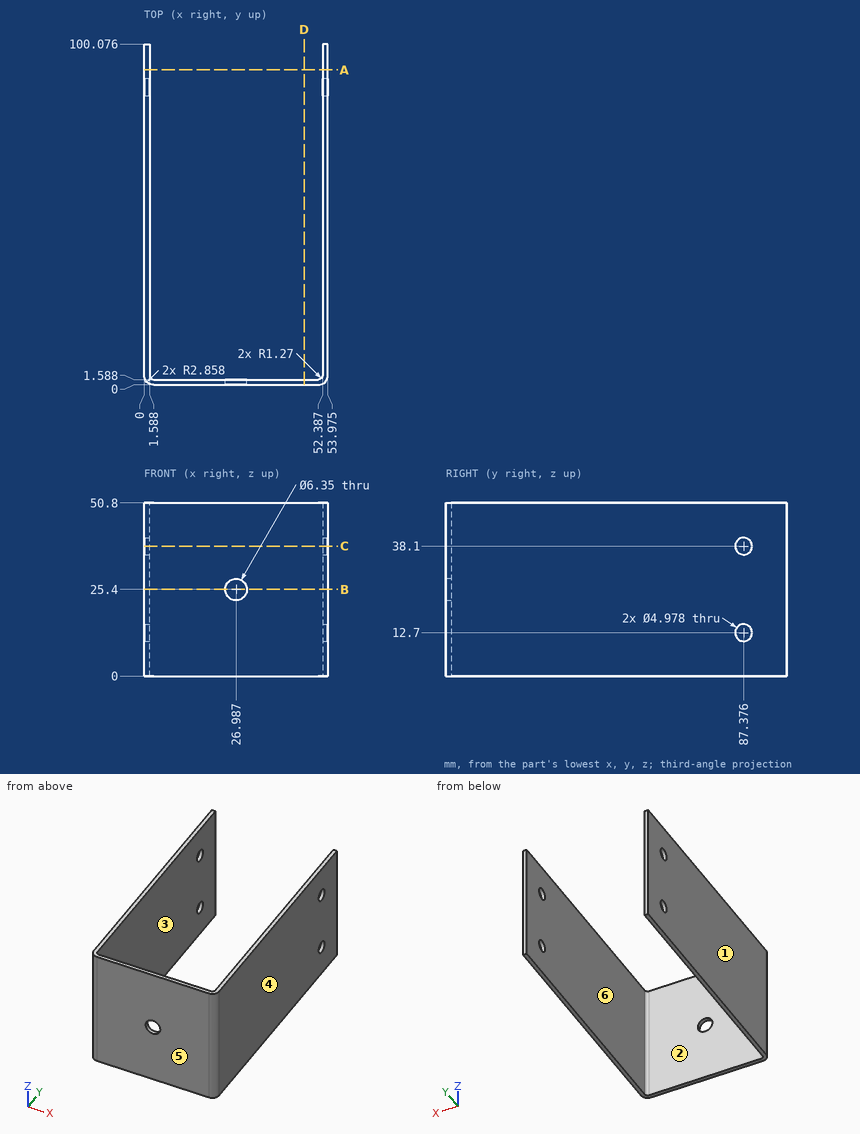
Print and shaded views of the part. All mm, measured from the part's lowest x, y and z. A direction names the side the tool comes from. Round coordinates to 2 decimals unless told otherwise and drop trailing zeros. Write each loop counter-clockwise with the first axis right and the second up, starting at its lowest first coordinate (ties: lowest second). Pieces come first, ordered by that corner, then holes.
(1) Slice it at C-C, the plane z = 38.1. Write the cut outline in (x, y) (1 decimal).
(2) Mould opens along X. For the marked faces 3, 4, 5 and 6 say: pulls with the +X half, pulls with the -X half, needs draft (parallel to the pull), parting line crosses it, or undercut.
(3) Probe line 1 along X through (y, z) = (17, 13.5) (1 decimal); line 2 along Y through (x, z) = (25.5, 47.5). List the from-to ranges inside material, lowest first.
(4) 3-axis set-ups, long thin cutter, end or side, ignore diameter. For the marked faces 1 and 2: which of +Z, -Z, +X, -X, +Y, -Y reach the whole face in a straight line?
(5) Slice it at D-D, the plane x = 47. Write the cut outline in (y, z).
(6) Slice it at B-B, the plane z = 25.4. Write the cut outline in (x, y) (1 decimal).
(7) Drop flat-ended pins along their axis: P1, Ø24, axis at x = 23.5, z = 16.5, coming from the +Y side; P2, Ø12, axis at x = 8, z = 21.5, coming from the +Y side. Give the stop position or say it passes through.
(8) Slice it at A-A, the plane y = 92.5. Write the cut outline in (x, z) (1 decimal).
From the geometry:
1. outline: (0, 2.9) arc R2.9 ccw to (2.9, 0) - (51.1, 0) arc R2.9 ccw to (54, 2.9) - (54, 84.9) - (52.4, 84.9) - (52.4, 2.9) arc R1.3 cw to (51.1, 1.6) - (2.9, 1.6) arc R1.3 cw to (1.6, 2.9) - (1.6, 84.9) - (0, 84.9) - close; (0, 89.9) - (1.6, 89.9) - (1.6, 100.1) - (0, 100.1) - close; (52.4, 89.9) - (54, 89.9) - (54, 100.1) - (52.4, 100.1) - close
2. face 3: undercut
2. face 4: pulls with the +X half
2. face 5: needs draft
2. face 6: undercut
3. line 1: x = 0 to 1.6, 52.4 to 54
3. line 2: y = 0 to 1.59
4. face 1: +Z, -Z, -X, +Y, -Y
4. face 2: +Z, -Z, +Y
5. outline: (0, 0) - (1.59, 0) - (1.59, 50.8) - (0, 50.8) - close
6. outline: (0, 2.9) arc R2.9 ccw to (2.9, 0) - (23.8, 0) - (23.8, 1.6) - (2.9, 1.6) arc R1.3 cw to (1.6, 2.9) - (1.6, 100.1) - (0, 100.1) - close; (30.2, 0) - (51.1, 0) arc R2.9 ccw to (54, 2.9) - (54, 100.1) - (52.4, 100.1) - (52.4, 2.9) arc R1.3 cw to (51.1, 1.6) - (30.2, 1.6) - close
7. P1: stops at y = 1.59
7. P2: stops at y = 1.92
8. outline: (0, 0) - (1.6, 0) - (1.6, 50.8) - (0, 50.8) - close; (52.4, 0) - (54, 0) - (54, 50.8) - (52.4, 50.8) - close
